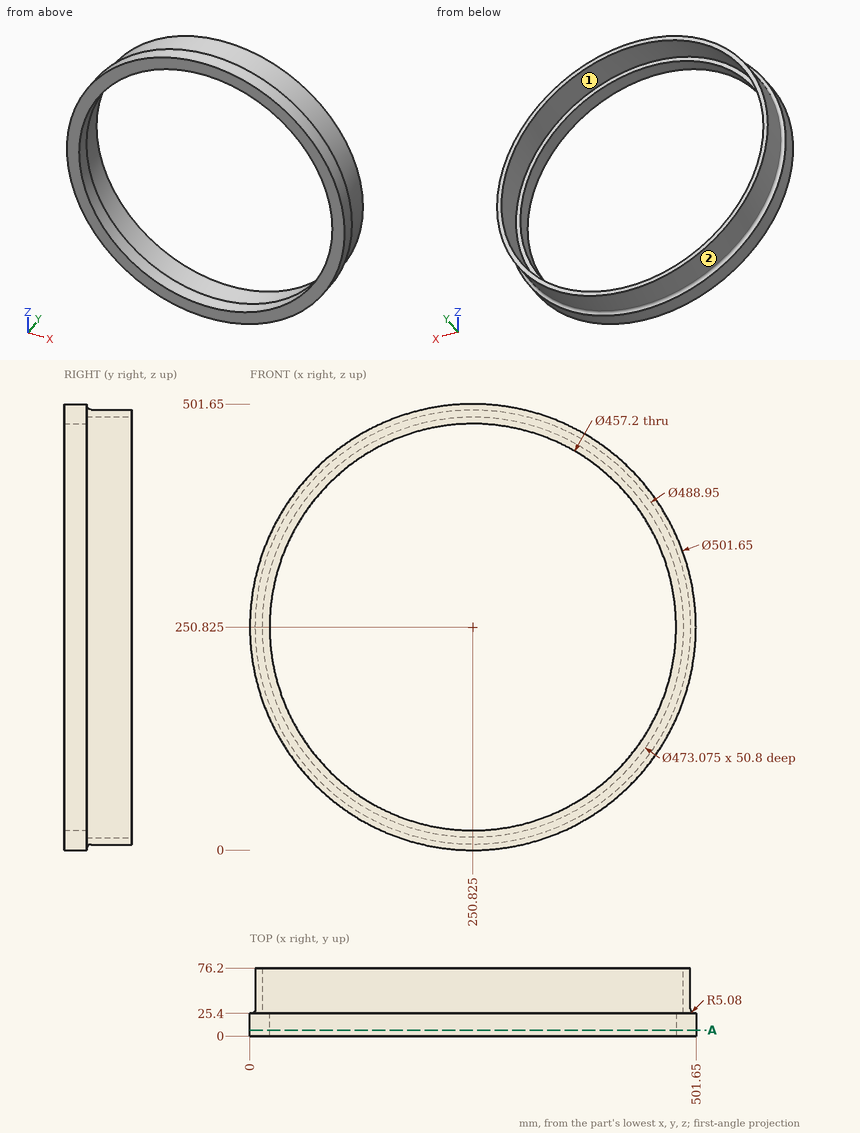
For this review, use the dimensioned drawing (mm, ordinates from the lowest corner) and the shaded views. Round coordinates to 2 decimals unless told otherwise and drop trailing zeros. Write each loop counter-clockwise with the first axis right and the second up, starting at its lowest first coordinate (ties: lowest second). Pieces come first, ordered by that corner, then holes. Notation, with made-up numbers: (-4, 54.5) -> (13, 54.5) arc R25 ccw to (13, 72.5) -> close; hole circle Ø3 at (83.25, 10). An arc over 180 degrees is marked (long way). Use CSV: the item, a comma, the result in double quotes.
Q1. Consider section A-A (y = 6.5). Give the boundary of the cut face in (x, z) (3 decimals), then the cut area to 3 significant figures.
Checks:
outline,"circle Ø501.65 at (250.825, 250.825); hole circle Ø457.2 at (250.825, 250.825)"
area,"33,500 mm²"
Q2. To check wall thickness, follow probe 1 along Z at (x, y) = (245.5, 51); probe 2 along X at (y, z) = (53, 331); probe 3 along X at (y, z) = (53, 373). State the ranges of each line that lie inside material, in increasing order. Write a range as [from, to].
Checks:
probe 1,"[6.41, 14.35], [487.3, 495.24]"
probe 2,"[19.87, 28.29], [473.36, 481.78]"
probe 3,"[39.07, 48.28], [453.37, 462.58]"
Q3. For pin 1 Ø1 at (x, y) = (394.5, 8) entering from +Z; pin 2 Ø5 at (x, y) = (60.5, 59.5) entering from +Z; pin 3 Ø2 at (y, z) = (16, 155) entering from +X, all flat-tipped, find the tip position at first contact; note any pin that passes through.
Checks:
pin 1,"z = 456.77"
pin 2,"z = 407.32"
pin 3,"x = 483.03"
Q4. Mouldability with a two-part tool opening along Z and no side actions: class the marked faces 1 and 2 as released by +Z, released by -Z, zero draft, split by the parting line, or undercut.
Checks:
face 1,"undercut"
face 2,"split by the parting line"
